from build123d import *

# Parameters (mm, degrees)
SALIENTE_EXTRUIR1_DEPTH     = 5
CROQUIS22_R                 = 1.475
CORTAR_EXTRUIR19_DEPTH      = 11.5
CROQUIS23_R                 = 1.475
CORTAR_EXTRUIR20_DEPTH      = 11.5
CORTAR_EXTRUIR21_DEPTH      = 36.958448256
CORTAR_EXTRUIR21_DEPTH_BACK = 36.958448256
CORTAR_EXTRUIR23_DEPTH      = 42.835511243
CORTAR_EXTRUIR23_DEPTH_BACK = 42.835511243
REDONDEO10_R                = 2.5
REDONDEO6_R                 = 1.5
CORTAR_EXTRUIR18_DEPTH      = 42.763006005
CORTAR_EXTRUIR18_DEPTH_BACK = 42.763006005
CROQUIS26_R                 = 1.175
SALIENTE_EXTRUIR2_DEPTH     = 11.5


with BuildPart() as part:
    # Croquis1 → Saliente-Extruir1 (new body)
    with BuildSketch(Plane.XY):
        with BuildLine():
            Line((-11.235063244, 0), (-5.235063244, 0))
            Line((-5.235063244, 0), (-5.235063244, 3))
            ThreePointArc((-5.235063244, 3), (-4.649276807, 4.414213562), (-3.235063244, 5))
            Line((-3.235063244, 5), (3.364936756, 5))
            ThreePointArc((3.364936756, 5), (4.779150318, 4.414213562), (5.364936756, 3))
            Line((5.364936756, 3), (5.364936756, 0))
            Line((5.364936756, 0), (13.264936756, 0))
            Line((13.264936756, 0), (13.264936756, 3))
            ThreePointArc((13.264936756, 3), (13.850723193, 4.414213562), (15.264936756, 5))
            Line((15.264936756, 5), (21.864936756, 5))
            ThreePointArc((21.864936756, 5), (23.279150318, 4.414213562), (23.864936756, 3))
            Line((23.864936756, 3), (23.864936756, 0))
            Line((23.864936756, 0), (29.864936756, 0))
            Line((29.864936756, 0), (29.864936756, -6))
            Line((29.864936756, -6), (23.864936756, -6))
            Line((23.864936756, -6), (23.864936756, -0.5))
            Line((23.864936756, -0.5), (12.364936756, -0.5))
            Line((12.364936756, -0.5), (12.364936756, -6))
            Line((12.364936756, -6), (5.364936756, -6))
            Line((5.364936756, -6), (5.364936756, -0.5))
            Line((5.364936756, -0.5), (-6.135063244, -0.5))
            Line((-6.135063244, -0.5), (-6.135063244, -6))
            Line((-6.135063244, -6), (-11.235063244, -6))
            Line((-11.235063244, -6), (-11.235063244, 0))
        make_face()
    extrude(amount=SALIENTE_EXTRUIR1_DEPTH)

    # Croquis22 → Cortar-Extruir19 (cut)
    with BuildSketch(Plane(origin=(5.364936756, 0, 0), x_dir=(0, 0, -1), z_dir=(1, 0, 0))):
        with Locations(Location((-2.5, 2.5, 0), (0, 0, 160.185071851))):
            Circle(CROQUIS22_R)
    extrude(amount=-CORTAR_EXTRUIR19_DEPTH, mode=Mode.SUBTRACT)

    # Croquis23 → Cortar-Extruir20 (cut)
    with BuildSketch(Plane(origin=(23.864936756, 0, 0), x_dir=(0, 0, -1), z_dir=(1, 0, 0))):
        with Locations(Location((-2.5, 2.5, 0), (0, 0, 160.185071851))):
            Circle(CROQUIS23_R)
    extrude(amount=-CORTAR_EXTRUIR20_DEPTH, mode=Mode.SUBTRACT)

    # Croquis24 → Cortar-Extruir21 (cut, two sides: drawn at the far end of the back side and taken through both)
    with BuildSketch(Plane(origin=(23.864936756, 0, 0), x_dir=(0, 0, -1), z_dir=(1, 0, 0)).offset(-CORTAR_EXTRUIR21_DEPTH_BACK)):
        with BuildLine():
            Line((-28.080519184, -19.184110571), (-5.642479376, 3.253929236))
            ThreePointArc((-5.642479376, 3.253929236), (-2.473578072, 4.566531134), (0.695323231, 3.253929236))
            Line((0.695323231, 3.253929236), (23.133363039, -19.184110571))
            Line((23.133363039, -19.184110571), (23.133363039, 44.280249847))
            Line((23.133363039, 44.280249847), (-28.080519184, 44.280249847))
            Line((-28.080519184, 44.280249847), (-28.080519184, -19.184110571))
        make_face()
    extrude(amount=CORTAR_EXTRUIR21_DEPTH + CORTAR_EXTRUIR21_DEPTH_BACK, mode=Mode.SUBTRACT)

    # Croquis28 → Cortar-Extruir23 (cut, two sides: drawn at the far end of the back side and taken through both)
    with BuildSketch(Plane(origin=(29.864936756, 0, 0), x_dir=(0, 0, -1), z_dir=(1, 0, 0)).offset(-CORTAR_EXTRUIR23_DEPTH_BACK)):
        with BuildLine():
            Line((-36.053555434, 5.476255779), (-5.598630977, -4.9471511))
            ThreePointArc((-5.598630977, -4.9471511), (-2.445331468, -5.471830492), (0.70796804, -4.9471511))
            Line((0.70796804, -4.9471511), (31.162892497, 5.476255779))
            Line((31.162892497, 5.476255779), (31.162892497, -58.902306946))
            Line((31.162892497, -58.902306946), (-36.053555434, -58.902306946))
            Line((-36.053555434, -58.902306946), (-36.053555434, 5.476255779))
        make_face()
    extrude(amount=CORTAR_EXTRUIR23_DEPTH + CORTAR_EXTRUIR23_DEPTH_BACK, mode=Mode.SUBTRACT)

    # Redondeo10
    # the kernel refuses this fillet: 2.5 mm, written as the material it takes off along each edge
    with BuildSketch(Plane(origin=(0.125968827, -5.13075911, 5), x_dir=(0, 1, 0), z_dir=(-1, 0, 0))) as redondeo10_piece_1:
        with BuildLine():
            CenterArc((2.159135079, 2.5), REDONDEO10_R, 180.432762449, 89.567237551)
            ThreePointArc((-0.340793609, 2.481117356), (-0.250491358, 1.229557299), (0, 0))
            Line((0, 0), (2.159135079, 0))
        make_face()
    extrude(amount=17.622064143, mode=Mode.SUBTRACT)
    with BuildSketch(Plane(origin=(0.210189755, -5.159802942, 0), x_dir=(0, 1, 0), z_dir=(-1, 0, 0))) as redondeo10_piece_2:
        with BuildLine():
            CenterArc((2.188178911, -2.5), REDONDEO10_R, 90, 90.432762449)
            ThreePointArc((-0.311749778, -2.518882644), (-0.238291712, -1.249240995), (0, 0))
            Line((0, 0), (2.188178911, 0))
        make_face()
    extrude(amount=17.790505999, mode=Mode.SUBTRACT)
    with BuildSketch(Plane(origin=(18.625968827, -5.13075911, 5), x_dir=(0, 1, 0), z_dir=(-1, 0, 0))) as redondeo10_piece_3:
        with BuildLine():
            CenterArc((2.159135079, 2.5), REDONDEO10_R, 180.432762449, 89.567237551)
            ThreePointArc((-0.340793609, 2.481117356), (-0.250491358, 1.229557299), (0, 0))
            Line((0, 0), (2.159135079, 0))
        make_face()
    extrude(amount=19.522064143, mode=Mode.SUBTRACT)
    with BuildSketch(Plane(origin=(18.710189755, -5.159802942, 0), x_dir=(0, 1, 0), z_dir=(-1, 0, 0))) as redondeo10_piece_4:
        with BuildLine():
            CenterArc((2.188178911, -2.5), REDONDEO10_R, 90, 90.432762449)
            ThreePointArc((-0.311749778, -2.518882644), (-0.238291712, -1.249240995), (0, 0))
            Line((0, 0), (2.188178911, 0))
        make_face()
    extrude(amount=19.690505999, mode=Mode.SUBTRACT)
    with BuildSketch(Plane(origin=(36.210189755, -5.159802942, 0), x_dir=(0, 1, 0), z_dir=(-1, 0, 0))) as redondeo10_piece_5:
        with BuildLine():
            CenterArc((2.188178911, -2.5), REDONDEO10_R, 90, 90.432762449)
            ThreePointArc((-0.311749778, -2.518882644), (-0.238291712, -1.249240995), (0, 0))
            Line((0, 0), (2.188178911, 0))
        make_face()
    extrude(amount=18.690505999, mode=Mode.SUBTRACT)
    with BuildSketch(Plane(origin=(36.125968827, -5.13075911, 5), x_dir=(0, 1, 0), z_dir=(-1, 0, 0))) as redondeo10_piece_6:
        with BuildLine():
            CenterArc((2.159135079, 2.5), REDONDEO10_R, 180.432762449, 89.567237551)
            ThreePointArc((-0.340793609, 2.481117356), (-0.250491358, 1.229557299), (0, 0))
            Line((0, 0), (2.159135079, 0))
        make_face()
    extrude(amount=18.522064143, mode=Mode.SUBTRACT)
    with BuildSketch(Plane(origin=(11.671123792, 3.786522656, 5), x_dir=(0, -1, 0), z_dir=(-1, 0, 0)), Plane(origin=(30.171123792, 3.786522656, 5), x_dir=(0, -1, 0), z_dir=(-1, 0, 0))) as redondeo10_piece_7:
        with BuildLine():
            CenterArc((1.720167689, -2.5), REDONDEO10_R, 90, 89.235979123)
            ThreePointArc((-0.779610048, -2.466664288), (-0.57165889, -1.175855696), (0, 0))
            Line((0, 0), (1.720167689, 0))
        make_face()
    extrude(amount=23.212374072, mode=Mode.SUBTRACT)
    with BuildSketch(Plane(origin=(11.789068224, 3.822043114, 0), x_dir=(0, -1, 0), z_dir=(-1, 0, 0)), Plane(origin=(30.289068224, 3.822043114, 0), x_dir=(0, -1, 0), z_dir=(-1, 0, 0))) as redondeo10_piece_8:
        with BuildLine():
            CenterArc((1.755688146, 2.5), REDONDEO10_R, 179.235979123, 90.764020877)
            ThreePointArc((-0.74408959, 2.533335712), (-0.562847764, 1.210625342), (0, 0))
            Line((0, 0), (1.755688146, 0))
        make_face()
    extrude(amount=23.448262936, mode=Mode.SUBTRACT)

    # Redondeo6
    redondeo6_edges = [part.edges().sort_by_distance(p)[0] for p in [
        (-11.235063244, 0, 2.5),
        (29.864936756, 0, 2.5),
    ]]
    fillet(redondeo6_edges, radius=REDONDEO6_R)

    # Croquis21 → Cortar-Extruir18 (cut, two sides: drawn at the far end of the back side and taken through both)
    with BuildSketch(Plane(origin=(29.864936756, 0, 0), x_dir=(0, 0, -1), z_dir=(1, 0, 0)).offset(-CORTAR_EXTRUIR18_DEPTH_BACK)):
        with BuildLine():
            Line((-36.990281352, 4.180822636), (-6.035224262, -4.762033155))
            ThreePointArc((-6.035224262, -4.762033155), (-2.696069768, -5.234705836), (0.643084727, -4.762033155))
            Line((0.643084727, -4.762033155), (31.598141816, 4.180822636))
            Line((31.598141816, 4.180822636), (31.598141816, -60.261096303))
            Line((31.598141816, -60.261096303), (-36.990281352, -60.261096303))
            Line((-36.990281352, -60.261096303), (-36.990281352, 4.180822636))
        make_face()
    extrude(amount=CORTAR_EXTRUIR18_DEPTH + CORTAR_EXTRUIR18_DEPTH_BACK, mode=Mode.SUBTRACT)

    # Croquis26 → Saliente-Extruir2 (add)
    with BuildSketch(Plane(origin=(-6.135063244, 0, 0), x_dir=(0, 0, -1), z_dir=(1, 0, 0))):
        with Locations(Location((-2.5, -3.45, 0), (0, 0, 180))):
            Circle(CROQUIS26_R)
    extrude(amount=SALIENTE_EXTRUIR2_DEPTH)


solid = part.part
Here's how the part is built. I have some questions about the finished solid (model axes, mm). A direction names the side the tool comes from. Coordinates: 2 decimals unless noted, no trailing zeros. Order: outer loops, then holes, each group sorted by start corner. A loop starts at its lowest first (then second) coordinate and runs counter-clockwise, first axis right, second up. Notation, with made-up numbers: (31.25, 57.5) - (55.25, 57.5) arc R27 cw to (55.25, 85.5) - close; hole circle Ø9 at (82, 84.25). An arc over 180 degrees is marked (long way). Use CSV: the item, a comma, the result in double quotes. Start each with the question number.
1. Please list where these lines run through material, in increasing order: line 1 (X direction, y = -4, z = 0.4); line 2 (X direction, y = -3, z = 2.8); line 3 (X direction, y = 2.5, z = 4.85). Write a range as from..to.
2. Suppose I cut it at A-A on z = 3.05. Give the number of separate pieces and of enclosed holes in the cut face, then the cut area to 3 significant figures.
3. Suppose I cut it at B-B on y = -3.45. List the corners of the cut face in (x, z) for me (3 decimals).
4. I'm going to push flat-ended pins straight in: pin 1 (1.3 mm diameter, centred on x = -8.5, z = 2, fed in from +Y); pin 2 (2.5 mm diameter, centred on y = 2, z = 2.5, fed in from +X); pin 3 (1.5 mm diameter, centred on y = 1.5, z = 3, fed in from -X); pin 4 (2.5 mm diameter, centred on y = 2.5, z = 2.5, fed in from +X). Where does each tip first touch, or does it pass through?
5. Suppose I cut it at C-C on x = -2.5. List the corners of the cut face in (y, z) for me (3 decimals).
6. For faces 1 (the face through (23.865, -3, 2)), 2 (the face through (4.95, 4.22, 2.47)), 3 (the face through (-0.47, -3.8, 3.62)), 4 (the face through (-5.235, 0.8, 2.5)), 5 (the face through (23.865, 0.85, 2.46)), which set-ups out of +Z, -Z, +X, -X, +Y, -Y let a thin tool reach every point of the face, with its end or its side?
7. Suppose I cut it at D-D on x = 19.5. List the corners of the cut face in (y, z) for me (3 decimals).
8. If we mould it in two halves opening along Y, with no side actions, what happens to faces 6 (the face through (5.365, -2, 2)), 7 (the face through (23.45, 4.22, 2.47)), 8 (the face through (8.914, -4.293, 4.622))? For each: +Y half, -Y half, draft (parallel to the pull), parting line (faces both ways), or undercut.
Output:
1,line 1,"x = -11.24..-6.14, 5.36..12.36, 23.86..29.86"
1,line 2,"x = -11.24..12.36, 23.86..29.86"
1,line 3,"x = -5.24..5.36, 13.26..23.86"
2,separate pieces,"3"
2,enclosed holes,"1"
2,area,"166 mm2"
3,outline,"(-11.235, 0.046) - (-6.135, 0.046) - (-6.135, 1.325) - (5.365, 1.325) - (5.365, 0.046) - (12.365, 0.046) - (12.365, 4.954) - (5.365, 4.954) - (5.365, 3.675) - (-6.135, 3.675) - (-6.135, 4.954) - (-11.235, 4.954) - close; (23.865, 0.046) - (29.865, 0.046) - (29.865, 4.954) - (23.865, 4.954) - close"
4,pin 1,"stops at y = 0"
4,pin 2,"stops at x = 23.86"
4,pin 3,"stops at x = -5.24"
4,pin 4,"passes through"
5,outline,"circle Ø2.35 at (-3.45, 2.5); (-0.5, 0) - (2.066, 0) arc R2.5 ccw to (2.066, 5) - (-0.5, 5) - close; hole circle Ø2.95 at (2.5, 2.5)"
6,face 1,"+Z, -Z, -Y"
6,face 2,"+Z, -Z, +Y"
6,face 3,"none"
6,face 4,"+Z, -Z, -X, +Y"
6,face 5,"+Z, -Z, +X, +Y"
7,outline,"(-0.5, 0) - (2.066, 0) arc R2.5 ccw to (2.066, 5) - (-0.5, 5) - close; hole circle Ø2.95 at (2.5, 2.5)"
8,face 6,"undercut"
8,face 7,"+Y half"
8,face 8,"-Y half"
